```python
from build123d import *

# Parameters (mm, degrees)
F0_W     = 20
F0_H     = 180
F1_DEPTH = 5
F2_R     = 3
F3_DEPTH = 5.001
F5_D     = 6
F7_D     = 6
F8_SIZE  = 0.5
F9_R     = 5


with BuildPart() as f1:
    # F0 (on Front) → F1 (new body)
    with BuildSketch(Plane.XZ):
        with Locations((10, 90)):
            Rectangle(F0_W, F0_H)
    extrude(amount=F1_DEPTH)

    # F2 (on face) → F3 (cut, through all)
    with BuildSketch(Plane.XZ.offset(5)):
        with Locations((10, 170)):
            Circle(F2_R)
    extrude(amount=-F3_DEPTH, mode=Mode.SUBTRACT)

    # F5 (through all)
    with Locations(Plane.XZ.offset(5)):
        with Locations((10, 70)):
            Hole(F5_D / 2)

    # F7 (through all)
    with Locations(Plane.XZ.offset(5)):
        with Locations((10, 10), (10, 20)):
            Hole(F7_D / 2)

    # F8
    f8_edges = [f1.edges().sort_by_distance(p)[0] for p in [
        (7, -5, 170),
        (7, 0, 170),
        (7, 0, 10),
        (7, 0, 20),
        (7, 0, 70),
        (7, -5, 10),
        (7, -5, 20),
        (7, -5, 70),
    ]]
    chamfer(f8_edges, length=F8_SIZE)

    # F9
    f9_edges = [f1.edges().sort_by_distance(p)[0] for p in [
        (20, -2.5, 180),
        (0, -2.5, 180),
    ]]
    fillet(f9_edges, radius=F9_R)


solid = f1.part
```
Input: part model. Units: mm. Frame: model coordinates. Give positions to 0.01 mm unless a question says otherwise; leave off trailing zeros. Order: outer loops, then holes, each group sorted by start corner. A loop starts at its lowest first (then second) coordinate and runs counter-clockwise, first axis right, second up. Notation, with made-up numbers: (65.25, 87) - (113.25, 87) arc R32 ccw to (113.25, 124) - close; hole circle Ø3 at (15, 26). An arc over 180 degrees is marked (long way). Use a Markdown table: item, result.
(1) Draft query along X for faces 1 (the cylindrical face through (12.4, -2.5, 8.2)), 2 (the flat face through (0, -2, 86)), 3 (the flat face through (20, -2, 86)), 4 (the flat face through (10, -2, 0)). Return one class per face: released by +X, released by -X, zero draft, split by the parting line, or undercut.
Computed values:
| item | result |
|---|---|
| face 1 | undercut |
| face 2 | released by -X |
| face 3 | released by +X |
| face 4 | zero draft |
(2) Line query: line 1 (Z direction, x = 10, y = -2.15); line 2 (X direction, y = -1.65, z = 170); line 3 (Z direction, x = 9, y = -3.2). Output: solid intervals per line, ascending. Write a range as from..to.
Computed values:
| item | result |
|---|---|
| line 1 | z = 0..7, 13..17, 23..67, 73..167, 173..180 |
| line 2 | x = 0..7, 13..20 |
| line 3 | z = 0..7.17, 12.83..17.17, 22.83..67.17, 72.83..167.17, 172.83..180 |
(3) Section query B-B (z = 70). Output: boundary loops of the cut face in (x, y).
Computed values:
| item | result |
|---|---|
| outline | (0, -5) - (6.5, -5) - (7, -4.5) - (7, -0.5) - (6.5, 0) - (0, 0) - close; (13, -4.5) - (13.5, -5) - (20, -5) - (20, 0) - (13.5, 0) - (13, -0.5) - close |
(4) Section query A-A (y = -2.55). Output: boundary loops of the cut face in (x, z), then the cut area to 3 significant figures.
Computed values:
| item | result |
|---|---|
| outline | (0, 0) - (20, 0) - (20, 175) arc R5 ccw to (15, 180) - (5, 180) arc R5 ccw to (0, 175) - close; hole circle Ø6 at (10, 10); hole circle Ø6 at (10, 20); hole circle Ø6 at (10, 70); hole circle Ø6 at (10, 170) |
| area | 3,480 mm2 |
(5) Section query C-C (x = 10). State how many separate pieces and enclosed holes the cut face has, then the cut area to 3 significant figures.
Computed values:
| item | result |
|---|---|
| separate pieces | 5 |
| enclosed holes | 0 |
| area | 778 mm2 |
